Verification items for the finished model (mm, model axes). A direction names the side the tool comes from. Give positions to 0.01 mm unless a question says otherwise; leave off trailing zeros. Return JSON: item names as keys, results as strings. Group by question number.
(1) Tool access check on faces 4 (the face through (-33.92, 47.01, 0.17)), 5 (the face through (-1, 60, 0)), 6 (the face through (-0.18, -49.23, -8.24)), 7 (the face through (36.6, 37.6, -8.2)), 8 (the face through (-30.1, 56.4, -6)). Record the directions out of +Z, -Z, +X, -X, +Y, -Y that give a thin tool (end or side, any length) a straight path to the whole face; none if there is none.
(2) Release check for a two-part mould opening along Y. For faces 1 (the face through (1, -60, 0)), 2 (the face through (-30.1, -45.6, -6)), 3 (the face through (-45, -1, 0)) record: pulls with the +Y half, pulls with the -Y half, needs draft (parallel to the pull), parting line crosses it, or undercut.
(3) Cross-section at A-A on z = 5. State how many separate pieces and enclosed holes the cut face has, then the cut area to 3 significant figures.
(4) Depth check by flat-ended pin: pin 1 Ø10.5 at (x, y) = (-36, 51) entering from -Z; pin 2 Ø2 at (y, z) = (-13, 7.5) entering from +X; pin 3 Ø5 at (x, y) = (28, 29.5) entering from -Z. Enter the tip coordinate at first touch or a pass-through.
(5) Thickness scan on line 1 along X through (y, z) = (-51, 1); line 2 along X through (y, z) = (-29, -4.5); line 3 along Y through (x, z) = (28, 4). Record the ranges inside material, lowest first.
from build123d import *

# Parameters (mm, degrees)
IZIM1_R                      = 4.5
Y_KSEKLIK_EKSTR_ZYON1_DEPTH  = 6.25
IZIM2_R                      = 40
Y_KSEKLIK_EKSTR_ZYON2_DEPTH  = 7.2
IZIM3_R                      = 10
KES_EKSTR_ZYON1_DEPTH        = 19.7
IZIM5_R                      = 5.1
IZIM5_R_2                    = 10
Y_KSEKLIK_EKSTR_ZYON4_DEPTH  = 3
RADYUS1_R                    = 1
M10_DI_LI_DELIK1_D           = 8.5
M10_DI_LI_DELIK1_DEPTH       = 16.5
M10_DI_LI_DELIK1_CSINK_D     = 10.05
M10_DI_LI_DELIK1_CSINK_ANGLE = 90
M10_DI_LI_DELIK1_TIP         = 2.553657631
IZIM8_R                      = 8
KES_EKSTR_ZYON2_DEPTH        = 0.5
IZIM9_R                      = 15
KES_EKSTR_ZYON3_DEPTH        = 12
IZIM12_W                     = 2
IZIM12_H                     = 5
PAH1_SIZE                    = 0.5


with BuildPart() as part:
    # Çizim1 → Yükseklik-Ekstrüzyon1 (new, symmetric)
    with BuildSketch(Plane.XY):
        with BuildLine():
            Line((36, -60), (-36, -60))
            ThreePointArc((-36, -60), (-42.363961031, -57.363961031), (-45, -51))
            Line((-45, -51), (-45, 51))
            ThreePointArc((-45, 51), (-42.363961031, 57.363961031), (-36, 60))
            Line((-36, 60), (36, 60))
            ThreePointArc((36, 60), (42.363961031, 57.363961031), (45, 51))
            Line((45, 51), (45, -51))
            ThreePointArc((45, -51), (42.363961031, -57.363961031), (36, -60))
        make_face()
        with Locations((-36, 51)):
            Circle(IZIM1_R, mode=Mode.SUBTRACT)
        with Locations((36, 51)):
            Circle(IZIM1_R, mode=Mode.SUBTRACT)
        with Locations((36, -51)):
            Circle(IZIM1_R, mode=Mode.SUBTRACT)
        with Locations((-36, -51)):
            Circle(IZIM1_R, mode=Mode.SUBTRACT)
    extrude(amount=Y_KSEKLIK_EKSTR_ZYON1_DEPTH, both=True)

    # Çizim2 → Yükseklik-Ekstrüzyon2 (add)
    with BuildSketch(Plane.XY.offset(6.25)):
        with Locations((0, 15.5)):
            Circle(IZIM2_R)
    extrude(amount=Y_KSEKLIK_EKSTR_ZYON2_DEPTH)

    # Çizim3 → Kes-Ekstrüzyon1 (cut)
    with BuildSketch(Plane.XY.offset(13.45)):
        with Locations((0, 15.5)):
            Circle(IZIM3_R)
    extrude(amount=-KES_EKSTR_ZYON1_DEPTH, mode=Mode.SUBTRACT)

    # Çizim5 → Yükseklik-Ekstrüzyon4 (add)
    # profile 1 of 5: a face of its own
    with BuildSketch(Plane(origin=(0, 0, -6.25), x_dir=(-1, 0, 0), z_dir=(0, 0, -1))):
        with BuildLine():
            ThreePointArc((-27.67613629, -40.470020932), (0.598697028, -49.232491897), (28.873530346, -40.470020932))
            ThreePointArc((28.873530346, -40.470020932), (29.909704021, -39.925668254), (31.044039725, -39.637123229))
            ThreePointArc((31.044039725, -39.637123229), (37.872111368, -35.981672207), (40.598697028, -28.732491897))
            Line((40.598697028, -28.732491897), (40.598697028, -27.538464678))
            ThreePointArc((40.598697028, -27.538464678), (40.778918063, -26.825594786), (41.276275007, -26.28402376))
            Line((41.276275007, -26.28402376), (42.598697028, -25.417032756))
            Line((42.598697028, -25.417032756), (42.598697028, 26.952048961))
            Line((42.598697028, 26.952048961), (41.276275007, 27.819039965))
            ThreePointArc((41.276275007, 27.819039965), (40.778918063, 28.360610991), (40.598697028, 29.073480884))
            Line((40.598697028, 29.073480884), (40.598697028, 30.267508103))
            ThreePointArc((40.598697028, 30.267508103), (37.872111368, 37.516688413), (31.044039725, 41.172139435))
            ThreePointArc((31.044039725, 41.172139435), (29.909704021, 41.46068446), (28.873530346, 42.005037137))
            ThreePointArc((28.873530346, 42.005037137), (0.598697028, 50.767508103), (-27.67613629, 42.005037137))
            ThreePointArc((-27.67613629, 42.005037137), (-28.712309964, 41.46068446), (-29.846645668, 41.172139435))
            ThreePointArc((-29.846645668, 41.172139435), (-36.674717311, 37.516688413), (-39.401302972, 30.267508103))
            Line((-39.401302972, 30.267508103), (-39.401302972, 29.073480884))
            ThreePointArc((-39.401302972, 29.073480884), (-39.581524007, 28.360610991), (-40.078880951, 27.819039965))
            Line((-40.078880951, 27.819039965), (-41.401302972, 26.952048961))
            Line((-41.401302972, 26.952048961), (-41.401302972, -25.417032756))
            Line((-41.401302972, -25.417032756), (-40.078880951, -26.28402376))
            ThreePointArc((-40.078880951, -26.28402376), (-39.581524007, -26.825594786), (-39.401302972, -27.538464678))
            Line((-39.401302972, -27.538464678), (-39.401302972, -28.732491897))
            ThreePointArc((-39.401302972, -28.732491897), (-36.674717311, -35.981672207), (-29.846645668, -39.637123229))
            ThreePointArc((-29.846645668, -39.637123229), (-28.712309964, -39.925668254), (-27.67613629, -40.470020932))
        make_face()
        with Locations((-28.401302972, 30.267508103)):
            Circle(IZIM5_R, mode=Mode.SUBTRACT)
        with Locations((29.598697028, 30.267508103)):
            Circle(IZIM5_R, mode=Mode.SUBTRACT)
        with Locations((-28.401302972, -28.732491897)):
            Circle(IZIM5_R, mode=Mode.SUBTRACT)
        with Locations((29.598697028, -28.732491897)):
            Circle(IZIM5_R, mode=Mode.SUBTRACT)
        with Locations(Location((0, 15.5, 0), (0, 0, 180))):
            Circle(IZIM5_R_2, mode=Mode.SUBTRACT)
    # profile 2 of 5: a face of its own
    with BuildSketch(Plane(origin=(0, 0, -6.25), x_dir=(-1, 0, 0), z_dir=(0, 0, -1))):
        with Locations((-28.401302972, -28.732491897)):
            Circle(IZIM5_R)
    # profile 3 of 5: a face of its own
    with BuildSketch(Plane(origin=(0, 0, -6.25), x_dir=(-1, 0, 0), z_dir=(0, 0, -1))):
        with Locations((29.598697028, -28.732491897)):
            Circle(IZIM5_R)
    # profile 4 of 5: a face of its own
    with BuildSketch(Plane(origin=(0, 0, -6.25), x_dir=(-1, 0, 0), z_dir=(0, 0, -1))):
        with Locations((29.598697028, 30.267508103)):
            Circle(IZIM5_R)
    # profile 5 of 5: a face of its own
    with BuildSketch(Plane(origin=(0, 0, -6.25), x_dir=(-1, 0, 0), z_dir=(0, 0, -1))):
        with Locations((-28.401302972, 30.267508103)):
            Circle(IZIM5_R)
    extrude(amount=Y_KSEKLIK_EKSTR_ZYON4_DEPTH)

    # Radyus1
    radyus1_edges = [part.edges().sort_by_distance(p)[0] for p in [
        (-0.598697028, -49.232491897, -6.25),
        (-29.909704021, -39.925668254, -6.25),
        (-37.872111368, -35.981672207, -6.25),
        (-40.598697028, -28.135478288, -6.25),
        (-40.778918063, -26.825594786, -6.25),
        (-41.937486018, -25.850528258, -6.25),
        (28.712309964, 41.46068446, -6.25),
        (36.674717311, 37.516688413, -6.25),
        (39.401302972, 29.670494493, -6.25),
        (39.581524007, 28.360610991, -6.25),
        (40.740091961, 27.385544463, -6.25),
        (41.401302972, 0.767508103, -6.25),
        (28.712309964, -39.925668254, -6.25),
        (36.674717311, -35.981672207, -6.25),
        (39.401302972, -28.135478288, -6.25),
        (39.581524007, -26.825594786, -6.25),
        (40.740091961, -25.850528258, -6.25),
        (-0.598697028, 50.767508103, -6.25),
        (-29.909704021, 41.46068446, -6.25),
        (-37.872111368, 37.516688413, -6.25),
        (-40.598697028, 29.670494493, -6.25),
        (-40.778918063, 28.360610991, -6.25),
        (-41.937486018, 27.385544463, -6.25),
        (-42.598697028, 0.767508103, -6.25),
    ]]
    fillet(radyus1_edges, radius=RADYUS1_R)

    # M10 Dişli Delik1
    with Locations(Plane(origin=(0, 0, -9.25), x_dir=(-1, 0, 0), z_dir=(0, 0, -1))):
        with Locations((-28, 29.5), (30, 29.5), (30, -29.5), (-28, -29.5)):
            CounterSinkHole(M10_DI_LI_DELIK1_D / 2, M10_DI_LI_DELIK1_CSINK_D / 2, depth=M10_DI_LI_DELIK1_DEPTH, counter_sink_angle=M10_DI_LI_DELIK1_CSINK_ANGLE)
            with Locations((0, 0, -(M10_DI_LI_DELIK1_DEPTH + M10_DI_LI_DELIK1_TIP / 2))):  # 118° drill point
                Cone(0, M10_DI_LI_DELIK1_D / 2, M10_DI_LI_DELIK1_TIP, mode=Mode.SUBTRACT)

    # Çizim8 → Kes-Ekstrüzyon2 (cut)
    with BuildSketch(Plane(origin=(0, 0, -6.25), x_dir=(-1, 0, 0), z_dir=(0, 0, -1))):
        with Locations((-36, -51)):
            Circle(IZIM8_R)
        with Locations((36, -51)):
            Circle(IZIM8_R)
        with Locations((36, 51)):
            Circle(IZIM8_R)
        with Locations((-36, 51)):
            Circle(IZIM8_R)
    extrude(amount=-KES_EKSTR_ZYON2_DEPTH, mode=Mode.SUBTRACT)

    # Çizim9 → Kes-Ekstrüzyon3 (cut)
    with BuildSketch(Plane.XY.offset(13.45)):
        with Locations((0, 15.5)):
            Circle(IZIM9_R)
    extrude(amount=-KES_EKSTR_ZYON3_DEPTH, mode=Mode.SUBTRACT)

    # Çizim12 → Kes-Döndür1 (revolve, cut)
    with BuildSketch(Plane(origin=(0, 0, 0), x_dir=(0, 0, -1), z_dir=(1, 0, 0)), mode=Mode.PRIVATE) as kes_d_nd_r1_sk:
        with Locations((-9.45, 29.965908827)):
            Rectangle(IZIM12_W, IZIM12_H)
    revolve(kes_d_nd_r1_sk.sketch.rotate(Axis((0, 15.5, -23.6616227), (0, 0, 1)), 270), axis=Axis((0, 15.5, -23.6616227), (0, 0, 1)), mode=Mode.SUBTRACT)

    # Pah1
    pah1_edges = [part.edges().sort_by_distance(p)[0] for p in [
        (-40, 15.5, 13.45),
    ]]
    chamfer(pah1_edges, length=PAH1_SIZE)


solid = part.part
Verdict:
{
 "1": {"face 4": "+Z, -Z", "face 5": "+Z, -Z, +X, -X, +Y", "face 6": "-Z, -Y", "face 7": "-Z, +X, +Y", "face 8": "-Z"},
 "2": {"face 1": "pulls with the -Y half", "face 2": "undercut", "face 3": "needs draft"},
 "3": {"separate pieces": "1", "enclosed holes": "9", "area": "9,540 mm²"},
 "4": {"pin 1": "z = -5.75", "pin 2": "x = 29.05", "pin 3": "z = 8.3"},
 "5": {"line 1": "-45 to -40.5, -31.5 to 31.5, 40.5 to 45", "line 2": "-45 to -34.22, -25.78 to 23.78, 32.22 to 45", "line 3": "-60 to -33.75, -25.25 to 25.25, 33.75 to 60"}
}
